For this review, use the dimensioned drawing (mm, ordinates from the lowest corner) and the shaded views. A direction names the side the tool comes from. Coordinates: 2 decimals unless noted, no trailing zeros. Loops run counter-clockwise (first coordinate to the right, second up) from the corner with the lowest first, then second, coordinate; pieces in that order, holes last. Notation, with made-up numbers: (89.5, 59.5) -> (99.5, 59.5) arc R25 ccw to (99.5, 76.5) -> close; hole circle Ø1 at (61.5, 16.25). An arc over 180 degrees is marked (long way). Answer as a JSON object with one key per item and string values.
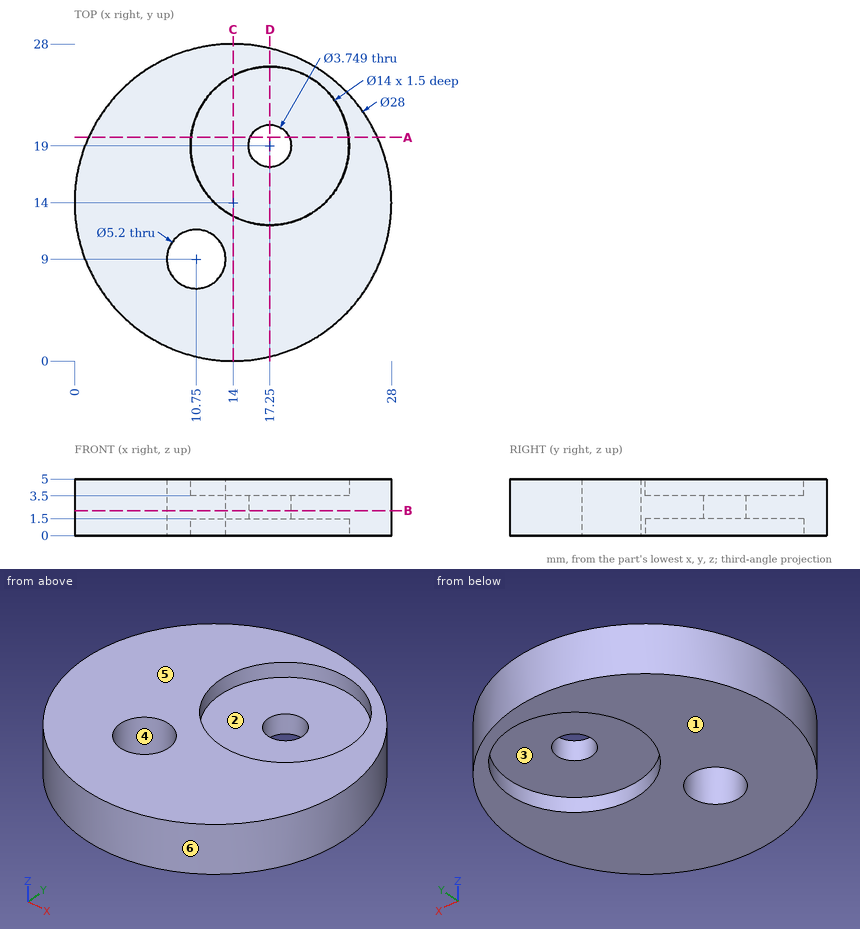
1) Add section C-C, the plane x = 14. Give the boundary of the cut face in (y, z).
Completed:
{"outline": "(0, 0) -> (12.8, 0) -> (12.8, 1.5) -> (25.2, 1.5) -> (25.2, 0) -> (28, 0) -> (28, 5) -> (25.2, 5) -> (25.2, 3.5) -> (12.8, 3.5) -> (12.8, 5) -> (0, 5) -> close"}
2) Clearance check with flat-ended pins moving along their axes: pin 1 Ø7 at (x, y) = (16, 19.5) entering from +Z; pin 2 Ø2 at (y, z) = (4.5, 2) entering from +X; pin 3 Ø3 at (y, z) = (22, 4) entering from -X. State where each tip first meets the part, or that it passes through.
Completed:
{"pin 1": "z = 3.5", "pin 2": "x = 25.12", "pin 3": "x = 1.6"}
3) Add section A-A, the plane y = 19.75. Give the boundary of the cut face in (x, z) (1 decimal), and give its area (3 significant figures).
Completed:
{"outline": "(1.2, 0) -> (10.3, 0) -> (10.3, 1.5) -> (15.5, 1.5) -> (15.5, 3.5) -> (10.3, 3.5) -> (10.3, 5) -> (1.2, 5) -> close; (19, 1.5) -> (24.2, 1.5) -> (24.2, 0) -> (26.8, 0) -> (26.8, 5) -> (24.2, 5) -> (24.2, 3.5) -> (19, 3.5) -> close", "area": "79.0 mm²"}
4) Add section B-B, the plane z = 2.2. Give the boundary of the cut face in (x, y).
Completed:
{"outline": "circle Ø28 at (14, 14); hole circle Ø5.2 at (10.75, 9); hole circle Ø3.75 at (17.25, 19)"}
5) For the marked faces 1, 2 and 3, list the 3-axis set-ups (+Z, -Z, +X, -X, +Y, -Y) from which the entire face can be reached by the end or side of a thin tool; tool diameter is ignored.
Completed:
{"face 1": "-Z, +X, -X, +Y, -Y", "face 2": "+Z", "face 3": "-Z"}
6) Add section D-D, the plane x = 17.25. Give the boundary of the cut face in (y, z).
Completed:
{"outline": "(0.38, 0) -> (12, 0) -> (12, 1.5) -> (17.13, 1.5) -> (17.13, 3.5) -> (12, 3.5) -> (12, 5) -> (0.38, 5) -> close; (20.87, 1.5) -> (26, 1.5) -> (26, 0) -> (27.62, 0) -> (27.62, 5) -> (26, 5) -> (26, 3.5) -> (20.87, 3.5) -> close"}
7) Wall thickness on probe 1 along Z at (x, y) = (22.5, 19.75); probe 2 along Y at (x, z) = (19.5, 0.8) (1 decimal); probe 3 along X at (y, z) = (10.5, 2.35) (1 decimal): over which ranges is each line inside the solid? List them lowest first.
Completed:
{"probe 1": "1.5 to 3.5", "probe 2": "1.1 to 12.4, 25.6 to 26.9", "probe 3": "0.4 to 8.6, 12.9 to 27.6"}
8) The part is to be moulded in two halves that separate along Y. For the marked faces 4, 5 and 6, say which applies: pulls with the +Y half, pulls with the -Y half, needs draft (parallel to the pull), parting line crosses it, or undercut.
Completed:
{"face 4": "undercut", "face 5": "needs draft", "face 6": "parting line crosses it"}
